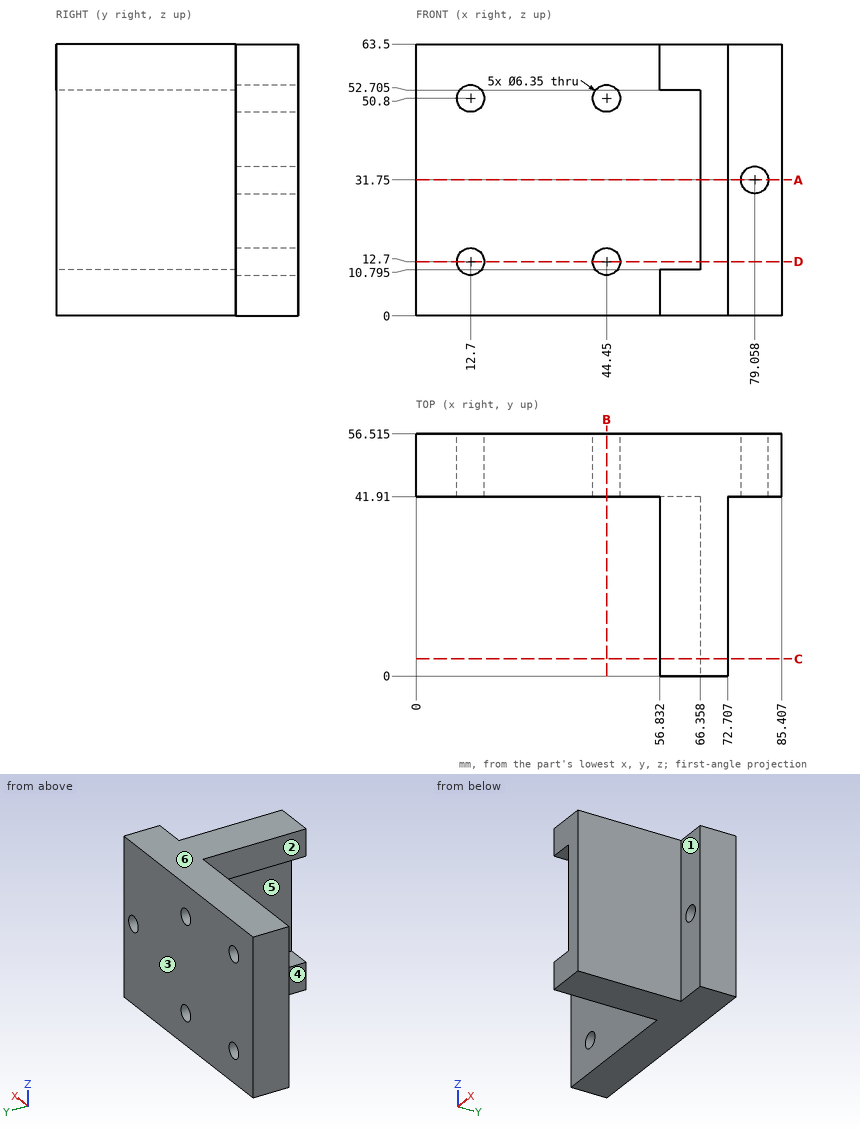
Geometry check sheet. Reference: drawing and pictorial views, mm from the part's lowest x, y, z. A direction names the side the tool comes from. Give positions to 0.01 mm unless a question says otherwise; leave off trailing zeros. Order: outer loops, then holes, each group sorted by start corner. A loop starts at its lowest first (then second) coordinate and runs counter-clockwise, first axis right, second up. Notation, with made-up numbers: (86.25, -2.75) - (109.25, -2.75) arc R26 ccw to (109.25, 21.25) - close; hole circle Ø7 at (-32.75, 31.25). An arc over 180 degrees is marked (long way). Answer as CSV lines item,"result". Start each with the question number.
Item 1: Section check B-B, the plane x = 44.45. Record the boundary of the cut face in (y, z) (1 decimal), plus the area to 3 significant figures.
Item 2: Access from +Z, -Z, +X, -X, +Y, -Y to the whole of each face (thin tool, end or side, straight path). Record for the marked faces 1, 2 and 3.
Item 3: Material ranges on L1, parallel to X at y = 49.5, z = 12.7 (1 decimal); L2, parallel to Z at x = 12.7, y = 51 (1 decimal); L3, parallel to X at y = 53, z = 50, recorded low to high.
Item 4: Mould release check, pull along Z, two halves, no side actions. Record for the marked faces 4, 5 and 6: released by +Z, released by -Z, zero draft, split by the parting line, or undercut.
Item 5: Gauge pin test, flat ends, axial feed: pin 1 (21 mm diameter, centred on y = 12, z = 25, fed in from -X); pin 2 (8.5 mm diameter, centred on x = 12.7, z = 12.7, fed in from -Y); pin 3 (12 mm diameter, centred on y = 12.5, z = 58.5, fed in from -X). Record the tip position at first contact, or that the pin passes through.
Item 6: Section check C-C, the plane y = 4. Record the boundary of the cut face in (x, z) (1 decimal).
Item 7: Section check D-D, the plane z = 12.7. Record the boundary of the cut face in (x, y) (1 decimal).
Item 8: Section check A-A, the plane z = 31.75. Record the boundary of the cut face in (x, y) (1 decimal), plus the area to 3 significant figures.
Filled in:
1,outline,"(41.9, 0) - (56.5, 0) - (56.5, 9.5) - (41.9, 9.5) - close; (41.9, 15.9) - (56.5, 15.9) - (56.5, 47.6) - (41.9, 47.6) - close; (41.9, 54) - (56.5, 54) - (56.5, 63.5) - (41.9, 63.5) - close"
1,area,"742 mm^2"
2,face 1,"+Z, -Z, +X, -Y"
2,face 2,"+Z, -Z, -X, -Y"
2,face 3,"+Z, -Z, +X, -X, +Y"
3,L1,"0 to 9.5, 15.9 to 41.3, 47.6 to 85.4"
3,L2,"0 to 9.5, 15.9 to 47.6, 54 to 63.5"
3,L3,"0 to 9.63, 15.77 to 41.38, 47.52 to 85.41"
4,face 4,"zero draft"
4,face 5,"undercut"
4,face 6,"released by +Z"
5,pin 1,"x = 66.36"
5,pin 2,"y = 41.91"
5,pin 3,"x = 56.83"
6,outline,"(56.8, 0) - (72.7, 0) - (72.7, 63.5) - (56.8, 63.5) - (56.8, 52.7) - (66.4, 52.7) - (66.4, 10.8) - (56.8, 10.8) - close"
7,outline,"(0, 41.9) - (9.5, 41.9) - (9.5, 56.5) - (0, 56.5) - close; (15.9, 41.9) - (41.3, 41.9) - (41.3, 56.5) - (15.9, 56.5) - close; (47.6, 41.9) - (66.4, 41.9) - (66.4, 0) - (72.7, 0) - (72.7, 41.9) - (85.4, 41.9) - (85.4, 56.5) - (47.6, 56.5) - close"
8,outline,"(0, 41.9) - (66.4, 41.9) - (66.4, 0) - (72.7, 0) - (72.7, 41.9) - (75.9, 41.9) - (75.9, 56.5) - (0, 56.5) - close; (82.2, 41.9) - (85.4, 41.9) - (85.4, 56.5) - (82.2, 56.5) - close"
8,area,"1,420 mm^2"
